Source: three-view drawing plus pictorial views. Frame: mm from the lowest corner of the part. A direction names the side the tool comes from. Give positions to 0.01 mm unless a question says otherwise; leave off trailing zeros. Order: outer loops, then holes, each group sorted by start corner. A loop starts at its lowest first (then second) coordinate and runs counter-clockwise, first axis right, second up. Notation, with made-up numbers: (-9, 46) - (43, 46) arc R23 cw to (43, 56) - close; hole circle Ø1 at (20, 66). An arc over 180 degrees is marked (long way). Use one line per item in the form item = value.
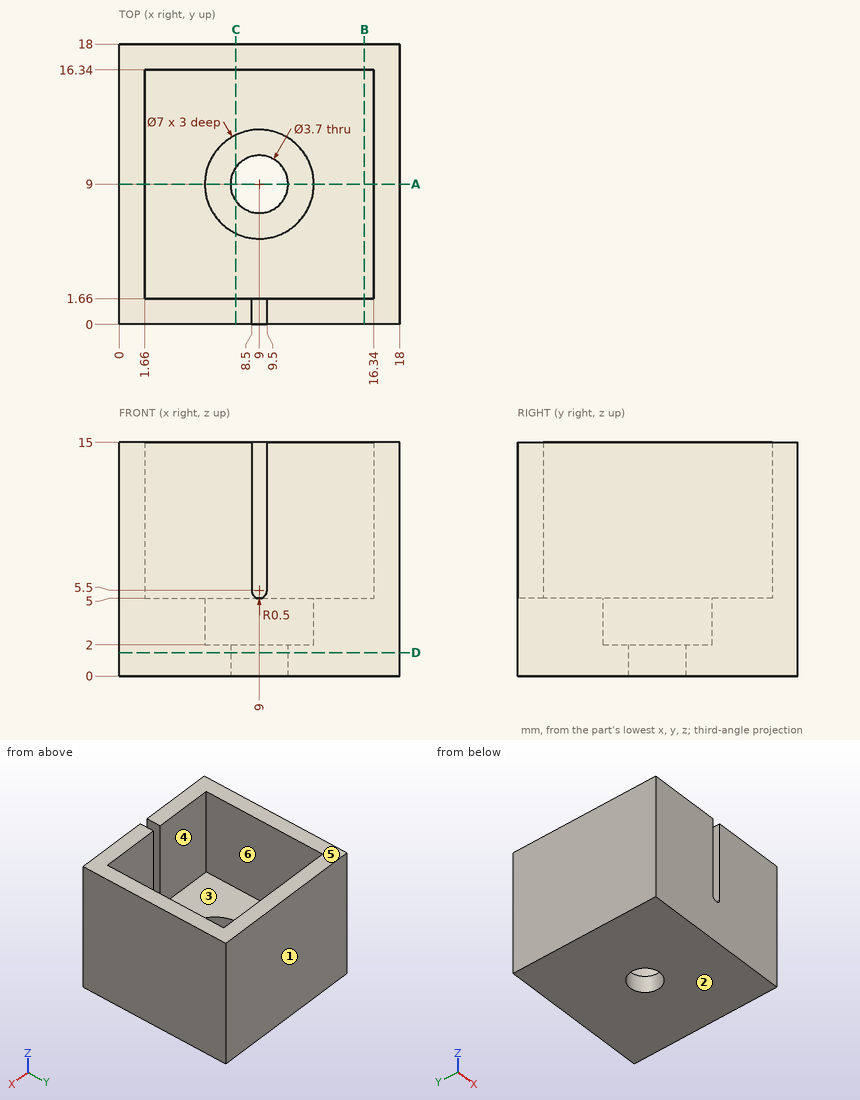
(1) Cut plane A-A on y = 9. Output: boundary loops of the cut face in (x, z).
Computed values:
outline = (0, 0) - (7.15, 0) - (7.15, 2) - (5.5, 2) - (5.5, 5) - (1.66, 5) - (1.66, 15) - (0, 15) - close; (10.85, 0) - (18, 0) - (18, 15) - (16.34, 15) - (16.34, 5) - (12.5, 5) - (12.5, 2) - (10.85, 2) - close
(2) Cut plane C-C on x = 7.5. Output: boundary loops of the cut face in (y, z), plus the area to 3 significant figures.
Computed values:
outline = (0, 0) - (7.92, 0) - (7.92, 2) - (5.84, 2) - (5.84, 5) - (1.66, 5) - (1.66, 15) - (0, 15) - close; (10.08, 0) - (18, 0) - (18, 15) - (16.34, 15) - (16.34, 5) - (12.16, 5) - (12.16, 2) - (10.08, 2) - close
area = 99.9 mm²
(3) Reachability of the marked faces 5 and 6 from +Z, -Z, +X, -X, +Y, -Y: full face, straight path, thin tool, end or side. Return the list, or none.
Computed values:
face_5 = +Z, +X, -X, +Y, -Y
face_6 = +Z
(4) Pull-direction query (Y, two-part tool) for the marked faces 1, 2, 3 and 4; classes: released by +Y, released by -Y, zero draft, split by the parting line, or undercut.
Computed values:
face_1 = released by +Y
face_2 = zero draft
face_3 = undercut
face_4 = undercut
(5) Cut plane D-D on z = 1.5. Output: boundary loops of the cut face in (x, y), plus the area to 3 significant figures.
Computed values:
outline = (0, 0) - (18, 0) - (18, 18) - (0, 18) - close; hole circle Ø3.7 at (9, 9)
area = 313 mm²
(6) Contact query for flat-ended pins moving along their axis: pin 1 Ø2 at (x, y) = (8.5, 10.5) entering from +Z; pin 2 Ø5 at (x, y) = (13, 13.5) entering from +Z. Output: stop coordinate, or through.
Computed values:
pin_1 = 2
pin_2 = 5
(7) Cut plane B-B on x = 15.75. Output: boundary loops of the cut face in (y, z), plus the area to 3 significant figures.
Computed values:
outline = (0, 0) - (18, 0) - (18, 15) - (16.34, 15) - (16.34, 5) - (1.66, 5) - (1.66, 15) - (0, 15) - close
area = 123 mm²
(8) Ray query, line 1 along X through (y, z) = (9, 0.7); line 2 along X through (y, z) = (9, 2.8). Return the intervals inside material, ascending.
Computed values:
line_1 = 0 to 7.15, 10.85 to 18
line_2 = 0 to 5.5, 12.5 to 18
